Build history of the part. All positions in model axes, mm. A direction names the side the tool comes from. Round coordinates to 2 decimals unless told otherwise and drop trailing zeros. Loops run counter-clockwise (first coordinate to the right, second up) from the corner with the lowest first, then second, coordinate; pieces in that order, holes last. Notation, with made-up numbers: (46.25, 41) -> (55.25, 41) arc R18 ccw to (55.25, 45) -> close; hole circle Ø8 at (52, 46.5). An arc over 180 degrees is marked (long way). Put each result on its own line as item: value. Start each with the question number.
Item 1: Flat gauge pins, fed straight in: pin 1 Ø6.5 at (x, z) = (9.5, 15) entering from +Y; pin 2 Ø11 at (x, z) = (22.5, 13) entering from -Y; pin 3 Ø1.5 at (y, z) = (20.5, 16) entering from +X. Where does each tip first touch, or does it go through?
Item 2: Drill centre lines: probe 1 along X at (y, z) = (35.25, 3.35); probe 2 along Y at (x, z) = (25, 7.25); probe 3 along X at (y, z) = (-1, 11). Where is each one in solid material? Low to high. Write a range as [from, to].
Item 3: Cut at B-B, the plane x = 21.5. List the corners of the cut face in (y, z), plus the area to 3 significant figures.
Item 4: Cut at D-D, the plane x = 12.5. List the corners of the cut face in (y, z), plus the area to 3 significant figures.
Item 5: Cut at A-A, the plane z = 3.35. List the corners of the cut face in (x, y).
Item 6: Pull direction Z, two halves, no side cores. Call faces 6 (the cylindrical face through (1.685, -0.194, 10.011)), 7 (the flat face through (25, 0, 11)), 8 (the flat face through (32, 14, 0)): +Z half, -Z half, draft (parallel to the pull), parting line (faces both ways), or undercut.
Item 7: Cut at C-C, the plane z = 11. List the corners of the cut face in (x, y).
Item 8: Tool access for faces 1 (the flat face through (5.95, -2, 11)), 2 (the flat face through (31.672, 18, 11)), 3 (the flat face through (34, 40, 11)), 4 (the cylindrical face through (26.324, 35.528, 3.262)), 5 (the flat face through (31.672, 39, 11)): list every direction of +Z, -Z, +X, -X, +Y, -Y with a clear straight run to the whole face (end or side of a thin tool).
Autodesk Inventor part; units mm, degrees
ref_plane "YZ Plane" through (0, 0, 0) normal (1, 0, 0) x (0, 1, 0)
ref_plane "XZ Plane" through (0, 0, 0) normal (0, 1, 0) x (-1, 0, 0)
ref_plane "XY Plane" through (0, 0, 0) normal (0, 0, 1) x (1, 0, 0)
sketch "Sketch1" plane through (0, 0, 0) normal (0, 0, 1) x (1, 0, 0)
  line L0 (0, 0) -> (50.1, 0)
  line L1 (50.1, 0) -> (50.1, 3)
  line L2 (50.1, 3) -> (0, 3)
  line L3 (0, 3) -> (0, 0)
  line L4 (35.6718, 0) -> (31.6718, 0)
  line L5 (31.6718, 0) -> (31.6718, 40)
  line L6 (31.6718, 40) -> (35.6718, 40)
  line L7 (35.6718, 40) -> (35.6718, 0)
  line L8 (31.6718, 37.5) -> (9.6718, 37.5)
  line L9 (9.6718, 37.5) -> (9.6718, 33.5)
  line L10 (9.6718, 33.5) -> (31.6718, 33.5)
  line L11 (31.6718, 33.5) -> (31.6718, 37.5)
  line L12 (5.95, 0) -> (44.15, 0)
  line L13 (44.15, 0) -> (44.15, 3)
  line L14 (44.15, 3) -> (5.95, 3)
  line L15 (5.95, 3) -> (5.95, 0)
  point P0 (35.6718, 3)
  point P1 (31.6718, 3)
  dimension "d0" = 50.1
  dimension "d1" = 3
  dimension "d2" = 40
  dimension "d3" = 22
  dimension "d4" = 4
  dimension "d5" = 2.5
  dimension "d6" = 38.2
  dimension "d7" = 5.95
  dimension "d30" = 4
extrude "Extrusion1" add sketch "Sketch1" along normal blind 22
sketch "Sketch2" plane through (0, 0, 0) normal (0, -1, 0) x (1, 0, 0)
  line L0 (50.1, 0) -> (50.1, 22)
  line L1 (0, 22) -> (50.1, 22)
  line L2 (50.1, 0) -> (44.15, 0)
  line L3 (44.15, 0) -> (44.15, 22)
  line L4 (44.15, 22) -> (50.1, 22)
  line L5 (50.1, 22) -> (50.1, 0)
  line L6 (0, 0) -> (5.95, 0)
  line L7 (5.95, 0) -> (5.95, 22)
  line L8 (5.95, 22) -> (0, 22)
  line L9 (0, 22) -> (0, 0)
  circle A0 centre (47.125, 11) radius 1.625
  circle A1 centre (2.975, 11) radius 1.625
  point P0 (47.125, 22)
  point P1 (0, 11)
  dimension "d10" = 5.95
  dimension "d11" = 5.95
  dimension "d14" = 3.25
  dimension "d15" = 3.25
  dimension "d16" = 2.975
  dimension "d17" = 11
  dimension "d18" = 2.975
  dimension "d19" = 11
extrude "Extrusion2" add sketch "Sketch2" along normal blind 3.3 contours L2 L3 L1 L0 | L7 L6 L9 L1 | A0 | A1
extrude "Extrusion3" cut sketch "Sketch2" along normal through all both and the other way through all contours A0 | A1
sketch "Sketch3" plane through (9.6718, 37.5, 0) normal (0, 1, 0) x (1, 0, 0)
  circle A0 centre (18.65, -18.65) radius 2
  circle A1 centre (18.65, -3.35) radius 2
  line L0 (22, 0) -> (22, -22)
  line L1 (22, -22) -> (-9.6718, -22)
  line L2 (22, 0) -> (0, 0)
  circle A2 centre (3.35, -3.35) radius 2
  line L3 (0, 0) -> (0, -22)
  point P0 (-9.6718, 0)
  point P1 (11, 0)
  dimension "d22" = 3.35
  dimension "d23" = 4
  dimension "d24" = 4
  dimension "d25" = 15.3
  dimension "d26" = 3.35
  dimension "d31" = 15.3
  dimension "d32" = 4
  dimension "d33" = 3.35
  dimension "d34" = 3.35
extrude "Extrusion4" cut sketch "Sketch3" against normal blind 10 contours A1 | A2
equation "\"d7\" = -0.5 * d6 + 0.5 * d0"
properties part number "IMU_shin_mount"
Reply:
1. pin 1: stops at y = 37.5
1. pin 2: stops at y = 0
1. pin 3: stops at x = 35.67
2. probe 1: x = [9.67, 11.02], [15.02, 26.32], [30.32, 35.67]
2. probe 2: y = [0, 3], [33.5, 37.5]
2. probe 3: x = [0, 1.35], [4.6, 5.95], [44.15, 45.5], [48.75, 50.1]
3. outline: (0, 0) -> (3, 0) -> (3, 22) -> (0, 22) -> close; (33.5, 0) -> (37.5, 0) -> (37.5, 22) -> (33.5, 22) -> close
3. area: 154 mm^2
4. outline: (0, 0) -> (3, 0) -> (3, 22) -> (0, 22) -> close; (33.5, 0) -> (37.5, 0) -> (37.5, 1.42) -> (33.5, 1.42) -> close; (33.5, 5.28) -> (37.5, 5.28) -> (37.5, 22) -> (33.5, 22) -> close
4. area: 139 mm^2
5. outline: (0, -3.3) -> (5.95, -3.3) -> (5.95, 0) -> (44.15, 0) -> (44.15, -3.3) -> (50.1, -3.3) -> (50.1, 3) -> (35.67, 3) -> (35.67, 40) -> (31.67, 40) -> (31.67, 37.5) -> (30.32, 37.5) -> (30.32, 33.5) -> (31.67, 33.5) -> (31.67, 3) -> (0, 3) -> close; (9.67, 33.5) -> (11.02, 33.5) -> (11.02, 37.5) -> (9.67, 37.5) -> close; (15.02, 33.5) -> (26.32, 33.5) -> (26.32, 37.5) -> (15.02, 37.5) -> close
6. face 6: undercut
6. face 7: draft
6. face 8: -Z half
7. outline: (0, -3.3) -> (1.35, -3.3) -> (1.35, 3) -> (0, 3) -> close; (4.6, -3.3) -> (5.95, -3.3) -> (5.95, 0) -> (44.15, 0) -> (44.15, -3.3) -> (45.5, -3.3) -> (45.5, 3) -> (35.67, 3) -> (35.67, 40) -> (31.67, 40) -> (31.67, 37.5) -> (9.67, 37.5) -> (9.67, 33.5) -> (31.67, 33.5) -> (31.67, 3) -> (4.6, 3) -> close; (48.75, -3.3) -> (50.1, -3.3) -> (50.1, 3) -> (48.75, 3) -> close
8. face 1: +Z, -Z, -Y
8. face 2: +Z, -Z, -X
8. face 3: +Z, -Z, +X, -X, +Y
8. face 4: +Y
8. face 5: +Z, -Z, -X, +Y
